Geometry check sheet. Reference: the model listing, model coordinates, mm. A direction names the side the tool comes from. Give positions to 0.01 mm unless a question says otherwise; leave off trailing zeros. Write each loop counter-clockwise with the first axis right and the second up, starting at its lowest first coordinate (ties: lowest second). Pieces come first, ordered by that corner, then holes.
(1) Thickness scan on line 1 along Y through (x, z) = (0, 47.5); line 2 along Z through (x, y) = (-3, 49); line 3 along Y through (x, z) = (0, 57). Record the ranges inside material, lowest first.
(2) Tool access check on faces 4 (the conical face through (-34.49, -10.86, 88.88)), 5 (the conical face through (5.524, 24.877, 49.195)), 6 (the flat face through (0, 15, 88.9)). Record the directions out of +Z, -Z, +X, -X, +Y, -Y that give a thin tool (end or side, any length) a straight path to the whole face; none if there is none.
(3) Cross-section at A-A (x = 0). Record the boundary of the cut face in (y, z) (3 decimals), and give its area (3 significant figures).
(4) Cross-section at D-D (z = 36). Record the boundary of the cut face in (x, y).
(5) Depth check by flat-ended pin: P1, Ø8, axis at y = 12, z = 57, coming from the +X side; P2, Ø1.5, axis at x = -30.5, z = 29.5, coming from the +Y side; P3, Ø10, axis at x = -39.5, y = 46, coming from the -Z side; P4, Ø2, axis at x = -6, z = 39, coming from the +Y side. Enter the tip coordinate at first touch or a pass-through.
(6) Cross-section at C-C (z = 83). Record the boundary of the cut face in (x, y) (3 decimals), and give its area (3 significant figures).
(7) Mould release check, pull along Y, two halves, no side actions. Record for faces 1 (the cylindrical face through (9.62, 7.38, 45.07)), 2 (the cylindrical face through (47.87, 36.71, 79.39)), 3 (the flat face through (49, 9, 18.561)): +Y half, -Y half, draft (parallel to the pull), parting line (faces both ways), or undercut.
```python
from build123d import *

# Parameters (mm, degrees)
F0_W        = 36.0753956601
F0_H        = 18.8608030145
F0_W_2      = 12.1251638026
F0_H_2      = 51.4777676715
F0_H_3      = 18.561429314
F2_C1_SIZE2 = 21.9075
F2_C1_SIZE  = 25.4
F2_C2_SIZE2 = 25.4
F2_C2_SIZE  = 21.9075
F4_SIZE2    = 25.4
F4_SIZE     = 0.41275


# Not quite as in the source:
# - a feature of the source that left no trace in its solid (it failed there, or was rolled back) is left out


with BuildPart() as f1:
    # F0 (on Front) → F1 (revolve)
    with BuildSketch(Plane.XZ):
        with Locations((-42.2873021699, 79.4695984927)):
            Rectangle(F0_W, F0_H)
        with Locations((-18.1870224386, 79.4695984927)):
            Rectangle(F0_W_2, F0_H)
        with Locations((-18.1870224386, 44.3003131497)):
            Rectangle(F0_W_2, F0_H_2)
        with Locations((-18.1870224386, 9.280714657)):
            Rectangle(F0_W_2, F0_H_3)
        with Locations((-42.2873021699, 9.280714657)):
            Rectangle(F0_W, F0_H_3)
    revolve(axis=Axis((0, 0, 53.2892593555), (0, 0, 1)))

    # F2: chamfer of 21.9075 x 25.4 on 2 edges, made by hand

    # F2_c1
    f2_c1_edges = [f1.edges().sort_by_distance(p)[0] for p in [
        (24.2496043399, 0, 70.0391969855),
    ]]
    f2_c1_side = f1.faces().sort_by_distance((24.6877543399, 0, 70.0391969855))[0]
    chamfer(f2_c1_edges, length=F2_C1_SIZE, length2=F2_C1_SIZE2, reference=f2_c1_side)

    # F2_c2
    f2_c2_edges = [f1.edges().sort_by_distance(p)[0] for p in [
        (24.2496043399, 0, 18.561429314),
    ]]
    f2_c2_side = f1.faces().sort_by_distance((24.2496043399, 0, 18.999579314))[0]
    chamfer(f2_c2_edges, length=F2_C2_SIZE, length2=F2_C2_SIZE2, reference=f2_c2_side)

    # F4
    f4_edges = [f1.edges().sort_by_distance(p)[0] for p in [
        (60.325, 0, 88.9),
    ]]
    chamfer(f4_edges, length=F4_SIZE, length2=F4_SIZE2)


solid = f1.part
```
Reply:
1. line 1: y = -24.25 to -12.12, 12.12 to 24.25
1. line 2: z = 0 to 19.04, 69.56 to 88.67
1. line 3: y = -34.53 to -12.12, 12.12 to 34.53
2. face 4: +Z
2. face 5: none
2. face 6: +Z, +X, -X, +Y, -Y
3. outline: (-60.325, 0) - (-12.124, 0) - (-12.124, 88.9) - (-34.925, 88.9) - (-60.325, 88.487) - (-60.325, 70.039) - (-49.65, 70.039) - (-24.25, 48.132) - (-24.25, 40.469) - (-49.65, 18.561) - (-60.325, 18.561) - close; (12.124, 0) - (60.325, 0) - (60.325, 18.561) - (49.65, 18.561) - (24.25, 40.469) - (24.25, 48.132) - (49.65, 70.039) - (60.325, 70.039) - (60.325, 88.487) - (34.925, 88.9) - (12.124, 88.9) - close
3. area: 5,960 mm2
4. outline: circle Ø58.86 at (0, 0); hole circle Ø24.25 at (0, 0)
5. P1: stops at x = 37.44
5. P2: stops at y = 22.71
5. P3: stops at z = 0
5. P4: stops at y = 26.46
6. outline: circle Ø120.65 at (0, 0); hole circle Ø24.249 at (0, 0)
6. area: 11,000 mm2
7. face 1: undercut
7. face 2: parting line
7. face 3: draft
